Autodesk Inventor part; units mm, degrees
ref_plane "YZ Plane" through (0, 0, 0) normal (1, 0, 0) x (0, 1, 0)
ref_plane "XZ Plane" through (0, 0, 0) normal (0, 1, 0) x (-1, 0, 0)
ref_plane "XY Plane" through (0, 0, 0) normal (0, 0, 1) x (1, 0, 0)
sketch "Esquisse1" plane through (0, 0, 0) normal (0, 1, 0) x (-1, 0, 0)
  line L0 (10.5, 47) -> (-10.5, 47)
  line L1 (-15.5, 42) -> (-15.5, -42)
  line L2 (-10.5, -47) -> (10.5, -47)
  line L3 (15.5, -42) -> (15.5, 42)
  line L4 (15.5, 47) -> (-15.5, -47) construction
  line L5 (-15.5, 47) -> (15.5, -47) construction
  arc A0 (15.5, 42) -> (10.5, 47) centre (10.5, 42) ccw
  arc A1 (-10.5, 47) -> (-15.5, 42) centre (-10.5, 42) ccw
  arc A2 (-15.5, -42) -> (-10.5, -47) centre (-10.5, -42) ccw
  arc A3 (10.5, -47) -> (15.5, -42) centre (10.5, -42) ccw
  point P0 (0, 0)
  dimension "d0" = 31
  dimension "d1" = 94
  dimension "d2" = 5
sketch "Esquisse2" plane through (0, 0, 0) normal (0, 1, 0) x (-1, 0, 0)
  point P0 (0, 0)
extrude "Extrusion1" add sketch "Esquisse1" along normal blind 20
sketch "Esquisse3" plane through (0, 20, 0) normal (0, 1, 0) x (1, 0, 0)
  line L0 (-8, -44.5) -> (8, -44.5)
  line L1 (13, -39.5) -> (13, 39.5)
  line L2 (8, 44.5) -> (-8, 44.5)
  line L3 (-13, 39.5) -> (-13, -39.5)
  line L4 (-13, -44.5) -> (13, 44.5) construction
  line L5 (13, -44.5) -> (-13, 44.5) construction
  arc A0 (-13, -39.5) -> (-8, -44.5) centre (-8, -39.5) ccw
  arc A1 (-8, 44.5) -> (-13, 39.5) centre (-8, 39.5) ccw
  arc A2 (13, 39.5) -> (8, 44.5) centre (8, 39.5) ccw
  arc A3 (8, -44.5) -> (13, -39.5) centre (8, -39.5) ccw
  circle A4 centre (0, 30) radius 1.5
  line L6 (-13, 0) -> (13, 0)
  circle A5 centre (0, -30) radius 1.5
  point P0 (0, 0)
  dimension "d5" = 26
  dimension "d6" = 89
  dimension "d7" = 5
  dimension "d10" = 3
  dimension "d11" = 30
extrude "Extrusion2" cut sketch "Esquisse3" against normal blind 17 contours A0 L3 L6 L1 A3 L0 | L3 A1 L2 A2 L1 L6 | A4 | A5
extrude "Extrusion3" cut sketch "Esquisse3" against normal blind 20 contours A4 | A5
chamfer "Chanfrein1" distance 2 angle 45 2 edges at (-1.5, 3, -30) (-1.5, 3, 30)
fillet "Congé1" radius 2 8 edges at (-15.5, 20, 0) (-14.0355, 20, 45.5355) (0, 20, 47) (14.0355, 20, 45.5355) (15.5, 20, 0) (14.0355, 20, -45.5355) (0, 20, -47) (-14.0355, 20, -45.5355)
properties part number "Support"
For this review, take the finished solid that the model builds, in its own axes (mm). A direction names the side the tool comes from. Round coordinates to 2 decimals unless told otherwise and drop trailing zeros. Write each loop counter-clockwise with the first axis right and the second up, starting at its lowest first coordinate (ties: lowest second). Pieces come first, ordered by that corner, then holes. Notation, with made-up numbers: (35.25, -20) - (41.25, -20) arc R22 cw to (41.25, 2) - close; hole circle Ø4 at (44.25, 40.25). An arc over 180 degrees is marked (long way). Use a Markdown table: item, result.
Q1. Machinability: for faces 5 (the cylindrical face through (-14.9, 19.43, 0.59)), 6 (the flat face through (-13, 12, -1)), which of the approach directions +Z, -Z, +X, -X, +Y, -Y give a long, thin tool a straight path to every point of the face, cutting with its end or side? Answer none if there is none.
Derived:
| item | result |
|---|---|
| face 5 | +Z, -Z, -X, +Y |
| face 6 | +Y |
Q2. Clearance check with a flat-ended pin moving along its axis: pin 1 (2 mm diameter, centred on x = 5.5, z = -5, fed in from +Y). State where the tip first meets the part, or that it passes through.
Derived:
| item | result |
|---|---|
| pin 1 | stops at y = 3 |
Q3. The part is to be moulded in two halves that separate along X. For faces 1 (the cylindrical face through (11.5, 11.62, 43.07)), 2 (the cylindrical face through (-14.07, 8.87, -45.5)), 3 (the flat face through (13, 12, 1)), 4 (the flat face through (0, 0, 1)), say which applies: pulls with the +X half, pulls with the -X half, needs draft (parallel to the pull), parting line crosses it, or undercut.
Derived:
| item | result |
|---|---|
| face 1 | undercut |
| face 2 | pulls with the -X half |
| face 3 | undercut |
| face 4 | needs draft |
Q4. We need section A-A (y = 6). Give the boundary of the cut face in (x, z).
Derived:
| item | result |
|---|---|
| outline | (-15.5, -42) arc R5 ccw to (-10.5, -47) - (10.5, -47) arc R5 ccw to (15.5, -42) - (15.5, 42) arc R5 ccw to (10.5, 47) - (-10.5, 47) arc R5 ccw to (-15.5, 42) - close; hole (-13, -39.5) arc R5 ccw to (-8, -44.5) - (8, -44.5) arc R5 ccw to (13, -39.5) - (13, 39.5) arc R5 ccw to (8, 44.5) - (-8, 44.5) arc R5 ccw to (-13, 39.5) - close |
Q5. Wall thickness on line 1 along Z through (x, y) = (0, 0.65); line 2 along X through (y, z) = (0.65, -30); line 3 along X through (y, z) = (15, 38.5): over which ranges is each line inside the solid? List them lowest first.
Derived:
| item | result |
|---|---|
| line 1 | z = -47 to -31.5, -28.5 to 28.5, 31.5 to 47 |
| line 2 | x = -15.5 to -1.5, 1.5 to 15.5 |
| line 3 | x = -15.5 to -13, 13 to 15.5 |
Q6. We need section B-B (x = 0). Give the boundary of the cut face in (y, z), plus the area to 3 significant figures.
Derived:
| item | result |
|---|---|
| outline | (0, -47) - (18, -47) arc R2 ccw to (20, -45) - (20, -44.5) - (3, -44.5) - (3, -33.5) - (1, -31.5) - (0, -31.5) - close; (0, -28.5) - (1, -28.5) - (3, -26.5) - (3, 26.5) - (1, 28.5) - (0, 28.5) - close; (0, 31.5) - (1, 31.5) - (3, 33.5) - (3, 44.5) - (20, 44.5) - (20, 45) arc R2 ccw to (18, 47) - (0, 47) - close |
| area | 339 mm2 |
Q7. We need section D-D (z = 11.5). Give the boundary of the cut face in (x, y), plus the area to 3 significant figures.
Derived:
| item | result |
|---|---|
| outline | (-15.5, 0) - (15.5, 0) - (15.5, 18) arc R2 ccw to (13.5, 20) - (13, 20) - (13, 3) - (-13, 3) - (-13, 20) - (-13.5, 20) arc R2 ccw to (-15.5, 18) - close |
| area | 176 mm2 |
Q8. We need section C-C (z = 30). Give the boundary of the cut face in (x, y).
Derived:
| item | result |
|---|---|
| outline | (-15.5, 0) - (-1.5, 0) - (-1.5, 1) - (-3.5, 3) - (-13, 3) - (-13, 20) - (-13.5, 20) arc R2 ccw to (-15.5, 18) - close; (1.5, 0) - (15.5, 0) - (15.5, 18) arc R2 ccw to (13.5, 20) - (13, 20) - (13, 3) - (3.5, 3) - (1.5, 1) - close |
